Input: part model. Units: mm. Frame: model coordinates. A direction names the side the tool comes from. Give positions to 0.01 mm unless a question says otherwise; leave off trailing zeros. One line per question, with ' | ' between items.
from build123d import *

# Parameters (mm, degrees)
SKETCH_1_W                = 200
SKETCH_1_H                = 48
HOLE_WIZARD_1_D           = 286
HOLE_WIZARD_1_DEPTH       = 15
SKETCH_4_W                = 134
SKETCH_4_H                = 10
SKETCH_5_W                = 7
SKETCH_5_H                = 8
HOLE_WIZARD_3_D           = 55
HOLE_WIZARD_3_CBORE_D     = 125
HOLE_WIZARD_3_CBORE_DEPTH = 19
CHAMFER_1_SIZE2           = 1.000000001
CHAMFER_1_SIZE            = 0.999999999
CHAMFER_2_SIZE            = 2.999999997
CHAMFER_2_SIZE2           = 3.000000003
CHAMFER_3_SIZE            = 13.999999987
CHAMFER_3_SIZE2           = 14.000000013
CHAMFER_4_SIZE            = 1.999999998
CHAMFER_4_SIZE2           = 2.000000002


with BuildPart() as part:
    # 草圖1 → 旋轉1 (revolve)
    with BuildSketch(Plane.XY, mode=Mode.PRIVATE) as revolve_1_sk:
        with Locations((100, 34)):
            Rectangle(SKETCH_1_W, SKETCH_1_H)
    revolve(revolve_1_sk.sketch.rotate(Axis((0, 58, 0), (0, -1, 0)), 270), axis=Axis((0, 58, 0), (0, -1, 0)))

    # 鑽孔1
    with Locations(Plane(origin=(0, 10, 0), x_dir=(-1, 0, 0), z_dir=(0, -1, 0))):
        with Locations((0, 0)):
            Hole(HOLE_WIZARD_1_D / 2, depth=HOLE_WIZARD_1_DEPTH)

    # 草圖4 → 旋轉2 (revolve)
    with BuildSketch(Plane.XY, mode=Mode.PRIVATE) as revolve_2_sk:
        with Locations((67, 20)):
            Rectangle(SKETCH_4_W, SKETCH_4_H)
    revolve(revolve_2_sk.sketch.rotate(Axis((0, 25, 0), (0, -1, 0)), 270), axis=Axis((0, 25, 0), (0, -1, 0)))

    # 草圖5 → 除料-旋轉1 (revolve, cut)
    with BuildSketch(Plane.XY, mode=Mode.PRIVATE) as cut_revolve_1_sk:
        with Locations((146.5, 14)):
            Rectangle(SKETCH_5_W, SKETCH_5_H)
    revolve(cut_revolve_1_sk.sketch.rotate(Axis((0, 18, 0), (0, -1, 0)), 270), axis=Axis((0, 18, 0), (0, -1, 0)), mode=Mode.SUBTRACT)

    # 鑽孔3 (through all)
    with Locations(Plane(origin=(0, 15, 0), x_dir=(-1, 0, 0), z_dir=(0, -1, 0))):
        with Locations((0, 0)):
            CounterBoreHole(HOLE_WIZARD_3_D / 2, HOLE_WIZARD_3_CBORE_D / 2, HOLE_WIZARD_3_CBORE_DEPTH)

    # 導角1
    chamfer_1_edges = [part.edges().sort_by_distance(p)[0] for p in [
        (62.5, 15, 0),
        (-27.5, 58, 0),
        (-27.5, 34, 0),
        (0, 58, 200),
    ]]
    chamfer(chamfer_1_edges, length=CHAMFER_1_SIZE, length2=CHAMFER_1_SIZE2)

    # 導角2
    chamfer_2_edges = [part.edges().sort_by_distance(p)[0] for p in [
        (0, 10, 150),
    ]]
    chamfer_2_side = [part.faces().sort_by_distance(p)[0] for p in [
        (0, 10, 194.343145751),
    ]]
    chamfer(chamfer_2_edges, length=CHAMFER_2_SIZE, length2=CHAMFER_2_SIZE2, reference=chamfer_2_side[0])

    # 導角3
    chamfer_3_edges = [part.edges().sort_by_distance(p)[0] for p in [
        (0, 10, 200),
    ]]
    chamfer_3_side = [part.faces().sort_by_distance(p)[0] for p in [
        (0, 10, 158.656854247),
    ]]
    chamfer(chamfer_3_edges, length=CHAMFER_3_SIZE, length2=CHAMFER_3_SIZE2, reference=chamfer_3_side[0])

    # 導角4
    chamfer_4_edges = [part.edges().sort_by_distance(p)[0] for p in [
        (-143, 18, 0),
    ]]
    chamfer_4_side = [part.faces().sort_by_distance(p)[0] for p in [
        (0, 18, 145.757359313),
    ]]
    chamfer(chamfer_4_edges, length=CHAMFER_4_SIZE, length2=CHAMFER_4_SIZE2, reference=chamfer_4_side[0])


solid = part.part
1. Reachability of faces 1 (the flat face through (123, 18, -78)), 2 (the flat face through (-41, 58, -3)) from +Z, -Z, +X, -X, +Y, -Y: full face, straight path, thin tool, end or side. Return the list, or none.
Determined:
face 1: -Y | face 2: +Z, -Z, +X, -X, +Y
2. Pull-direction query (Z, two-part tool) for faces 3 (the conical face through (56.13, 10.88, -178.25)), 4 (the cylindrical face through (-5.961, 46.154, 26.846)), 5 (the flat face through (-151, 10, 27)); classes: pulls with the +Z half, pulls with the -Z half, needs draft (parallel to the pull), parting line crosses it, or undercut.
Determined:
face 3: parting line crosses it | face 4: undercut | face 5: needs draft
3. Pin query (flat end, axial travel): P1, Ø8, axis at x = -79, z = -51, coming from the -Y side; P2, Ø12, axis at y = 52.5, z = -96.5, coming from the -X side; P3, Ø4, axis at x = 146, y = 24.5, coming from the +Z side. Return the tip coordinate at first contact, or that it passes through.
Determined:
P1: stops at y = 15 | P2: stops at x = -178.35 | P3: stops at z = 138.79
4. Ray query, line 1 along X through (y, z) = (28, 0); line 2 along Z through (x, y) = (41, 19); line 3 along X through (y, z) = (47, 0). Return the intervals inside material, ascending. Write a range as from..to.
Determined:
line 1: x = -200..-62.5, 62.5..200 | line 2: z = -190.64..-138.04, -127.57..-47.17, 47.17..127.57, 138.04..190.64 | line 3: x = -200..-27.5, 27.5..200
